Autodesk Inventor part; units mm, degrees
ref_plane "YZ Plane" through (0, 0, 0) normal (1, 0, 0) x (0, 1, 0)
ref_plane "XZ Plane" through (0, 0, 0) normal (0, 1, 0) x (-1, 0, 0)
ref_plane "XY Plane" through (0, 0, 0) normal (0, 0, 1) x (1, 0, 0)
sketch "Boceto1" plane through (0, 0, 0) normal (0, 0, 1) x (1, 0, 0)
  line L0 (0, 0) -> (25, 0)
  line L1 (25, 0) -> (25, 24)
  line L2 (25, 24) -> (0, 24)
  line L3 (0, 24) -> (0, 0)
  circle A0 centre (2, 2) radius 1.05
  circle A1 centre (23, 2) radius 1.05
  circle A2 centre (2, 14.5) radius 1.05
  circle A3 centre (23, 14.5) radius 1.05
  line L4 (0, 17) -> (25, 17)
  line L5 (0, 0) -> (25, 0)
  line L6 (25, 0) -> (25, -5)
  line L7 (25, -5) -> (0, -5)
  line L8 (0, -5) -> (0, 0)
  dimension "d0" = 25
  dimension "d1" = 24
  dimension "d2" = 2.1
  dimension "d3" = 2
  dimension "d4" = 2
  dimension "d7" = 21
  dimension "d10" = 12.5
  dimension "d13" = 7
  dimension "d14" = 5
extrude "Extrusión1" add sketch "Boceto1" along normal blind 3 contours L3 L4 L1 L0 | L0 L6 L7 L8
properties part number "Sujetador_camara"
Check sheet for the modelled part. Datum: model origin and axes. Units: mm. Give positions to 0.01 mm unless a question says otherwise; leave off trailing zeros. Loops run counter-clockwise (first coordinate to the right, second up) from the corner with the lowest first, then second, coordinate; pieces in that order, holes last. Notation, with made-up numbers: (38, -24) - (88, -24) arc R16 ccw to (88, 4) - close; hole circle Ø9 at (30.5, 4). An arc over 180 degrees is marked (long way). One line per question, with ' | ' between items. Start each with the question number.
1. Cross-section at A-A, the plane z = 1.25. Enter the section's corners in (x, y), plus the area to 3 significant figures.
2. Cross-section at B-B, the plane y = 14.5. Enter the section's corners in (x, z), plus the area to 3 significant figures.
3. Cross-section at C-C, the plane x = 2. Enter the section's corners in (y, z).
4. Material ranges on line 1 along Y through (x, z) = (2, 0.8); line 2 along X through (y, z) = (1.75, 2.7), recorded low to high. Write a range as [from, to].
5. Draft check along Y on faces 1 (the flat face through (13, -5, 1)), 2 (the flat face through (12, 17, 1)), 3 (the flat face through (25, 6, 1)), 4 (the cylindrical face through (2.485, 2.932, 1.479)). Enter one of: released by +Y, released by -Y, zero draft, split by the parting line, or undercut.
Check result:
1) outline: (0, -5) - (25, -5) - (25, 17) - (0, 17) - close; hole circle Ø2.1 at (2, 2); hole circle Ø2.1 at (2, 14.5); hole circle Ø2.1 at (23, 2); hole circle Ø2.1 at (23, 14.5) | area: 536 mm2
2) outline: (0, 0) - (0.95, 0) - (0.95, 3) - (0, 3) - close; (3.05, 0) - (21.95, 0) - (21.95, 3) - (3.05, 3) - close; (24.05, 0) - (25, 0) - (25, 3) - (24.05, 3) - close | area: 62.4 mm2
3) outline: (-5, 0) - (0.95, 0) - (0.95, 3) - (-5, 3) - close; (3.05, 0) - (13.45, 0) - (13.45, 3) - (3.05, 3) - close; (15.55, 0) - (17, 0) - (17, 3) - (15.55, 3) - close
4) line 1: y = [-5, 0.95], [3.05, 13.45], [15.55, 17] | line 2: x = [0, 0.98], [3.02, 21.98], [24.02, 25]
5) face 1: released by -Y | face 2: released by +Y | face 3: zero draft | face 4: undercut
